The listing builds one solid part. Answer for the finished solid, in the listing's coordinates (mm). A direction names the side the tool comes from. Round coordinates to 2 decimals unless told otherwise and drop trailing zeros. Write each loop counter-clockwise with the first axis right and the second up, starting at its lowest first coordinate (ties: lowest second). Pieces come first, ordered by that corner, then holes.
from build123d import *

# Parameters (mm, degrees)
SKETCH1_W                       = 25.4
SKETCH1_H                       = 25.4
SKETCH1_W_2                     = 19.05
SKETCH1_H_2                     = 19.05
BOSS_EXTRUDE1_DEPTH             = 292.1
F_10_CLEARANCE_HOLE1_D          = 5.1054
CUT_EXTRUDE1_REACH              = 296.3
SKETCH6_R                       = 9.525
CUT_EXTRUDE1_DIRECTION_2_DEPTH  = 295.300407747
F_4_CLEARANCE_HOLE1_D           = 3.2639
F_4_CLEARANCE_HOLE1_CSINK_D     = 4.5339
F_4_CLEARANCE_HOLE1_CSINK_ANGLE = 90
F_10_CLEARANCE_HOLE2_D          = 5.1054


with BuildPart() as part:
    # Sketch1 → Boss-Extrude1 (new body)
    with BuildSketch(Plane.XY):
        with Locations((-12.7, 12.7)):
            Rectangle(SKETCH1_W, SKETCH1_H)
        with Locations((-12.7, 12.7)):
            Rectangle(SKETCH1_W_2, SKETCH1_H_2, mode=Mode.SUBTRACT)
    extrude(amount=BOSS_EXTRUDE1_DEPTH)

    # #10 Clearance Hole1 (through all)
    with Locations(Plane(origin=(0, 25.4, 0), x_dir=(1, 0, 0), z_dir=(0, 1, 0))):
        with Locations((-12.7, -254), (-12.7, -241.3), (-12.7, -228.6)):
            Hole(F_10_CLEARANCE_HOLE1_D / 2)

    # Cut-Extrude1: up to this face of the body (flat: up to its plane)
    cut_extrude1_end = Plane(part.part.faces().sort_by_distance((0, 12.7, 146.05))[0])
    # Sketch6 → Cut-Extrude1 (cut, up to the picked face)
    with BuildSketch(Plane.ZY.offset(25.4), mode=Mode.PRIVATE) as cut_extrude1_sk1:
        with Locations(Location((241.3, 12.711043767, 0), (0, 0, 87.24065676))):
            Circle(SKETCH6_R)
    cut_extrude1_tool1 = split(extrude(cut_extrude1_sk1.sketch, amount=-CUT_EXTRUDE1_REACH, mode=Mode.PRIVATE), bisect_by=cut_extrude1_end, keep=Keep.BOTH, mode=Mode.PRIVATE)
    # Sketch6 → Cut-Extrude1 (cut, up to the picked face)
    with BuildSketch(Plane.ZY.offset(25.4), mode=Mode.PRIVATE) as cut_extrude1_sk2:
        with Locations(Location((34.925, 12.711043767, 0), (0, 0, 270))):
            Circle(SKETCH6_R)
    cut_extrude1_tool2 = split(extrude(cut_extrude1_sk2.sketch, amount=-CUT_EXTRUDE1_REACH, mode=Mode.PRIVATE), bisect_by=cut_extrude1_end, keep=Keep.BOTH, mode=Mode.PRIVATE)
    add(cut_extrude1_tool1.solids().sort_by(Axis((-25.4, 12.711044, 241.3), (1, 0, 0)))[0], mode=Mode.SUBTRACT)
    add(cut_extrude1_tool2.solids().sort_by(Axis((-25.4, 12.711044, 34.925), (1, 0, 0)))[0], mode=Mode.SUBTRACT)

    # Sketch6 → Cut-Extrude1 direction 2 (cut)
    with BuildSketch(Plane.ZY.offset(25.4)):
        with Locations(Location((241.3, 12.711043767, 0), (0, 0, 87.24065676))):
            Circle(SKETCH6_R)
        with Locations(Location((34.925, 12.711043767, 0), (0, 0, 270))):
            Circle(SKETCH6_R)
    extrude(amount=CUT_EXTRUDE1_DIRECTION_2_DEPTH, mode=Mode.SUBTRACT)

    # #4 Clearance Hole1 (through all)
    with Locations(Plane(origin=(0, 25.4, 0), x_dir=(1, 0, 0), z_dir=(0, 1, 0))):
        with Locations((-9.525, -6.35), (-15.875, -6.35)):
            CounterSinkHole(F_4_CLEARANCE_HOLE1_D / 2, F_4_CLEARANCE_HOLE1_CSINK_D / 2, counter_sink_angle=F_4_CLEARANCE_HOLE1_CSINK_ANGLE)

    # #10 Clearance Hole2 (through all)
    with Locations(Plane(origin=(0, 25.4, 0), x_dir=(1, 0, 0), z_dir=(0, 1, 0))):
        with Locations((-12.7, -50.8), (-12.7, -38.1), (-12.7, -25.4)):
            Hole(F_10_CLEARANCE_HOLE2_D / 2)


solid = part.part
1. Given pin 1 (3 mm diameter, centred on x = -12.7, z = 228.6, fed in from -Y) (3 decimals), flat-ended and moving along its own axis, determine where the tip first touches the part or whether it passes through.
Geometry says:
pin 1: passes through
2. For a pull along Y with two mould halves and no side action, classify faces 1 (the face through (-13, 0, 144)), 2 (the face through (-2, 13, 0)), 3 (the face through (-13, 3.175, 144)), 4 (the face through (-22.225, 13, 144)) as released by +Y, released by -Y, zero draft, split by the parting line, or undercut.
Geometry says:
face 1: released by -Y
face 2: zero draft
face 3: undercut
face 4: undercut
3. Section B-B on y = 15 is taken. Determine the outline of the cut face in (x, z) (3 decimals).
Geometry says:
outline: (-25.4, 0) - (-22.225, 0) - (-22.225, 25.679) - (-25.4, 25.679) - close; (-25.4, 44.171) - (-22.225, 44.171) - (-22.225, 232.054) - (-25.4, 232.054) - close; (-25.4, 250.546) - (-22.225, 250.546) - (-22.225, 292.1) - (-25.4, 292.1) - close; (-3.175, 0) - (0, 0) - (0, 25.679) - (-3.175, 25.679) - close; (-3.175, 44.171) - (0, 44.171) - (0, 232.054) - (-3.175, 232.054) - close; (-3.175, 250.546) - (0, 250.546) - (0, 292.1) - (-3.175, 292.1) - close
4. Straight lines are drawn through the part: line 1 along Z through (x, y) = (-23.5, 12); line 2 along X through (y, z) = (12.5, 50) (3 decimals); line 3 along Y through (x, z) = (-19, 101.5) (3 decimals). For each, find the intervals that lie inside material, in ascending order.
Geometry says:
line 1: z = 0 to 25.43, 44.42 to 231.8, 250.8 to 292.1
line 2: x = -25.4 to -22.225, -3.175 to 0
line 3: y = 0 to 3.175, 22.225 to 25.4
5. Section C-C on z = 38.1 is taken. Determine the outline of the cut face in (x, y) (3 decimals), plus the area to 3 significant figures.
Geometry says:
outline: (-25.4, 0) - (-15.253, 0) - (-15.253, 3.175) - (-22.225, 3.175) - (-22.225, 3.731) - (-25.4, 3.731) - close; (-25.4, 21.691) - (-22.225, 21.691) - (-22.225, 22.225) - (-15.253, 22.225) - (-15.253, 25.4) - (-25.4, 25.4) - close; (-10.147, 0) - (0, 0) - (0, 3.731) - (-3.175, 3.731) - (-3.175, 3.175) - (-10.147, 3.175) - close; (-10.147, 22.225) - (-3.175, 22.225) - (-3.175, 21.691) - (0, 21.691) - (0, 25.4) - (-10.147, 25.4) - close
area: 136 mm2
6. A tool of negligible diameter and unlimited length cuts with its end or side. For faces 5 (the face through (-13, 25.4, 144)), 6 (the face through (-3.175, 13, 144)), from which of +Z, -Z, +X, -X, +Y, -Y can it reach the whole face along a straight path? Write none if from no direction.
Geometry says:
face 5: +Z, -Z, +X, -X, +Y
face 6: +Z, -Z
7. Section A-A on z = 254 is taken. Determine the outline of the cut face in (x, y) (3 decimals).
Geometry says:
outline: (-25.4, 0) - (-15.253, 0) - (-15.253, 3.175) - (-22.225, 3.175) - (-22.225, 22.225) - (-15.253, 22.225) - (-15.253, 25.4) - (-25.4, 25.4) - close; (-10.147, 0) - (0, 0) - (0, 25.4) - (-10.147, 25.4) - (-10.147, 22.225) - (-3.175, 22.225) - (-3.175, 3.175) - (-10.147, 3.175) - close
